Geometry check sheet. Reference: the model listing, model coordinates, mm. A direction names the side the tool comes from. Coordinates: 2 decimals unless noted, no trailing zeros. Order: outer loops, then holes, each group sorted by start corner. A loop starts at its lowest first (then second) coordinate and runs counter-clockwise, first axis right, second up. Notation, with made-up numbers: (4.25, -36.5) - (46.25, -36.5) arc R8 cw to (46.25, -32.5) - close; hole circle Ø11 at (-1.5, -0.75). An arc over 180 degrees is marked (long way). Use CSV: the item, a comma, the result in double quotes. Start each with the question number.
1) Sectioned sample at B-B, the plane y = -9.5. Record the cut outline in (x, z), and give its area (3 significant figures).
2) Tool access check on faces 4 (the flat face through (245.014, -10, -120)), 5 (the flat face through (290, -7, -268)). Record the directions out of +Z, -Z, +X, -X, +Y, -Y that give a thin tool (end or side, any length) a straight path to the whole face; none if there is none.
3) Thickness scan on probe 1 along X at (y, z) = (-9.75, -147). Record the ranges inside material, lowest first. Write a range as [from, to].
4) Sectioned sample at A-A, the plane x = 260. Record the cut outline in (y, z), and give its area (4 significant figures).
5) Draft check along Z on faces 1 (the flat face through (0, -7, -268)), 2 (the cylindrical face through (260, -10, -55)), 3 (the flat face through (143, -7, -529)). Enter one of: released by +Z, released by -Z, zero draft, split by the parting line, or undercut.
from build123d import *

# Parameters (mm, degrees)
F0_W     = 290
F0_H     = 529
F1_DEPTH = 15
F3_DEPTH = 10


with BuildPart() as f1:
    # F0 (on Front) → F1 (new body)
    with BuildSketch(Plane.XZ):
        with Locations((145, -264.5)):
            Rectangle(F0_W, F0_H)
    extrude(amount=F1_DEPTH)

    # F2 (on face) → F3 (cut)
    with BuildSketch(Plane.XZ.offset(15)):
        with BuildLine():
            Line((245.0136655844, -169.3598587771), (245.0136655844, -170.6401412229))
            ThreePointArc((245.0136655844, -170.6401412229), (260.3201435355, -184.9965832147), (275, -170))
            ThreePointArc((275, -170), (260.3201435355, -155.0034167853), (245.0136655844, -169.3598587771))
        make_face()
        with BuildLine():
            ThreePointArc((245.0136655844, -169.3598587771), (260.3201435355, -155.0034167853), (275, -170))
            Line((275.0000000457, -170), (274.9922312187, -70.4827039319))
            ThreePointArc((274.9922312187, -70.4827039319), (260.0787738422, -84.9997931546), (245.0136655844, -70.6401412229))
            Line((245.0136655844, -70.6401412229), (245.0136655844, -169.3598587771))
        make_face()
        with BuildLine():
            ThreePointArc((245.0136655844, -70.6401412229), (260.0787738422, -84.9997931546), (274.9922312187, -70.4827039319))
            Line((274.9922312187, -70.4827039319), (274.9921556713, -69.5149553341))
            ThreePointArc((274.9921556713, -69.5149553341), (259.4373995265, -55.0105543562), (245.0136655844, -70.6401412229))
        make_face()
    extrude(amount=-F3_DEPTH, mode=Mode.SUBTRACT)


solid = f1.part
Evaluation:
1,outline,"(0, -529) - (290, -529) - (290, 0) - (0, 0) - close; hole (245.01, -170.64) arc R15 ccw to (275, -170) - (274.99, -69.51) arc R15 ccw (long way) to (245.01, -70.64) - close"
1,area,"150,000 mm²"
2,face 4,"-Y"
2,face 5,"+Z, -Z, +X, +Y, -Y"
3,probe 1,"[0, 245.01], [275, 290]"
4,outline,"(-15, -529) - (0, -529) - (0, 0) - (-15, 0) - (-15, -55) - (-5, -55) - (-5, -185) - (-15, -185) - close"
4,area,"6,635 mm²"
5,face 1,"zero draft"
5,face 2,"undercut"
5,face 3,"released by -Z"
